```python
from build123d import *

# Parameters (mm, degrees)
SKETCH1_R           = 6.01
SKETCH1_W           = 6.3
SKETCH1_H           = 6.3
BOSS_EXTRUDE1_DEPTH = 5.5
BOSS_EXTRUDE2_START = 2
SKETCH1_3_R         = 8
SKETCH1_3_R_2       = 6.01
SKETCH1_3_W         = 6.3
SKETCH1_3_H         = 6.3
BOSS_EXTRUDE2_DEPTH = 2
FILLET1_R           = 0.5


with BuildPart() as part:
    # Sketch1 → Boss-Extrude1 (new body)
    with BuildSketch(Plane.XY):
        Circle(SKETCH1_R)
        Rectangle(SKETCH1_W, SKETCH1_H, mode=Mode.SUBTRACT)
    extrude(amount=-BOSS_EXTRUDE1_DEPTH)

    # Sketch1_3 → Boss-Extrude2 (add)
    # profile 1 of 2: a face of its own
    with BuildSketch(Plane.XY.offset(BOSS_EXTRUDE2_START)):
        Circle(SKETCH1_3_R)
        Circle(SKETCH1_3_R_2, mode=Mode.SUBTRACT)
    # profile 2 of 2: a face of its own
    with BuildSketch(Plane.XY.offset(BOSS_EXTRUDE2_START)):
        Circle(SKETCH1_3_R_2)
        Rectangle(SKETCH1_3_W, SKETCH1_3_H, mode=Mode.SUBTRACT)
    extrude(amount=-BOSS_EXTRUDE2_DEPTH)

    # Fillet1
    fillet1_edges = [part.edges().sort_by_distance(p)[0] for p in [
        (-8, 0, 0),
        (-6.01, 0, -5.5),
    ]]
    fillet(fillet1_edges, radius=FILLET1_R)


solid = part.part
```
Can you work these out from the model? Positions are in its coordinate system, mm. A direction names the side the tool comes from. Coordinates: 2 decimals unless noted, no trailing zeros. Loops run counter-clockwise (first coordinate to the right, second up) from the corner with the lowest first, then second, coordinate; pieces in that order, holes last.
1) Imagine slicing it at C-C on z = 1.5. List the corners of the cut face in (x, y) for me, plus the area to 3 significant figures.
2) Imagine slicing it at D-D on z = -2.25. List the corners of the cut face in (x, y) for me, plus the area to 3 significant figures.
3) Thinking about a two-plate mould opening in Y: for faces 1 (the flat face through (-3.15, 0, -2)), 2 (the flat face through (3.15, 0, -2)), 3 (the flat face through (3.4, 0.1, 2)), 4 (the cylindrical face through (5.73, 1.81, -2.46)), which applies, pulls with the +Y half, pulls with the -Y half, needs draft (parallel to the pull), parting line crosses it, or undercut?
4) Imagine slicing it at A-A on y = 0. List the corners of the cut face in (x, z) for me, plus the area to 3 significant figures.
5) Which directions (+Z, -Z, +X, -X, +Y, -Y) give clear straight access to the entire face, cutting with the end or side of a thin tool? Please do faces 5 (the flat face through (0, 3.15, -2)), 6 (the flat face through (0, -4, -5.5)), 7 (the flat face through (-6, 2, 0)).
6) For pin 1 (1 mm diameter, centred on x = 1.5, z = -1.5, fed in from -Y); pin 2 (3 mm diameter, centred on y = 1.5, z = -3, fed in from -X); pin 3 (8 mm diameter, centred on x = 1.5, y = 5.5, fed in from -Z); pin 4 (3 mm diameter, centred on x = -4, z = -3.5, fed in from +Y), each with a flat end and sliding along its axis, tell me the tip position at first contact or that it passes through.
7) I need wall thicknesses on probe 1 along Y at (x, z) = (-0.25, 0.75); probe 2 along X at (y, z) = (-0.25, -2.5); probe 3 along Y at (x, z) = (0, -2.25). Which ranges of each line are inside material? Lowest first, please.
Completed:
1. outline: circle Ø16 at (0, 0); hole (-3.15, -3.15) - (3.15, -3.15) - (3.15, 3.15) - (-3.15, 3.15) - close
1. area: 161 mm2
2. outline: circle Ø12.02 at (0, 0); hole (-3.15, -3.15) - (3.15, -3.15) - (3.15, 3.15) - (-3.15, 3.15) - close
2. area: 73.8 mm2
3. face 1: undercut
3. face 2: undercut
3. face 3: needs draft
3. face 4: parting line crosses it
4. outline: (-8, 0.5) arc R0.5 ccw to (-7.5, 0) - (-6.01, 0) - (-6.01, -5) arc R0.5 ccw to (-5.51, -5.5) - (-3.15, -5.5) - (-3.15, 2) - (-8, 2) - close; (3.15, -5.5) - (5.51, -5.5) arc R0.5 ccw to (6.01, -5) - (6.01, 0) - (7.5, 0) arc R0.5 ccw to (8, 0.5) - (8, 2) - (3.15, 2) - close
4. area: 50.6 mm2
5. face 5: +Z, -Z
5. face 6: -Z, +X, -X, +Y, -Y
5. face 7: -Z
6. pin 1: stops at y = -5.93
6. pin 2: stops at x = -6.01
6. pin 3: stops at z = -5.5
6. pin 4: stops at y = 5.47
7. probe 1: y = -8 to -3.15, 3.15 to 8
7. probe 2: x = -6 to -3.15, 3.15 to 6
7. probe 3: y = -6.01 to -3.15, 3.15 to 6.01
